The listing builds one solid part. Answer for the finished solid, in the listing's coordinates (mm). Face numbers are marked on the shaded views. A direction names the side the tool comes from. Give positions to 0.01 mm unless a question says otherwise; leave off trailing zeros. Order: outer loops, then holes, each group sorted by start corner. A loop starts at its lowest first (then second) coordinate and runs counter-clockwise, first axis right, second up. Notation, with made-up numbers: (27.25, 60) - (44.25, 60) arc R22 ccw to (44.25, 80) - close; hole circle Ø1 at (-4, 48). An arc over 180 degrees is marked (long way). Answer in a Markdown table with one row per item.
from build123d import *

# Parameters (mm, degrees)
F0_R     = 14.95
F1_DEPTH = 20.6
F2_R     = 12.5
F3_DEPTH = 4
F4_R     = 12.5
F5_DEPTH = 4.5
F6_R     = 5
F7_DEPTH = 25


with BuildPart() as f1:
    # F0 (on Front) → F1 (new body)
    with BuildSketch(Plane.XZ):
        Circle(F0_R)
    extrude(amount=F1_DEPTH)

    # F2 (on face) → F3 (join)
    with BuildSketch(Plane.XZ.offset(20.6)):
        Circle(F2_R)
    extrude(amount=F3_DEPTH)

    # F4 (on face) → F5 (cut)
    with BuildSketch(Plane(origin=(0, 0, 0), x_dir=(-1, 0, 0), z_dir=(0, 1, 0))):
        Circle(F4_R)
    extrude(amount=-F5_DEPTH, mode=Mode.SUBTRACT)

    # F6 (on face) → F7 (cut)
    with BuildSketch(Plane(origin=(0, -4.5, 0), x_dir=(-1, 0, 0), z_dir=(0, 1, 0))):
        Circle(F6_R)
    extrude(amount=-F7_DEPTH, mode=Mode.SUBTRACT)


solid = f1.part
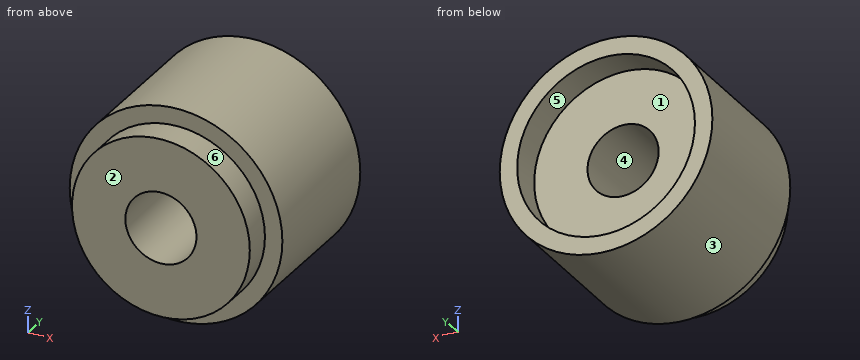
Item 1: Find section B-B on x = 0. Write down the section's boundary in (y, z).
Answer block:
| item | result |
|---|---|
| outline | (-24.6, -12.5) - (-20.6, -12.5) - (-20.6, -14.95) - (0, -14.95) - (0, -12.5) - (-4.5, -12.5) - (-4.5, -5) - (-24.6, -5) - close; (-24.6, 5) - (-4.5, 5) - (-4.5, 12.5) - (0, 12.5) - (0, 14.95) - (-20.6, 14.95) - (-20.6, 12.5) - (-24.6, 12.5) - close |
Item 2: Determine the mould class of the marked faces 1, 2 and 3 for opening direction X: pulls with the +X half, pulls with the -X half, needs draft (parallel to the pull), parting line crosses it, or undercut.
Answer block:
| item | result |
|---|---|
| face 1 | undercut |
| face 2 | needs draft |
| face 3 | parting line crosses it |
Item 3: Consider line 1 (Z direction, x = 0, y = -18.25); line 2 (Y direction, x = -10.5, z = -0.5); line 3 (Y direction, x = -9.5, z = -11). Determine where each line is inside the solid, lowest interval first.
Answer block:
| item | result |
|---|---|
| line 1 | -14.95 to -5, 5 to 14.95 |
| line 2 | -24.6 to -4.5 |
| line 3 | -20.6 to 0 |
Item 4: Find section A-A on z = 0. Write down the section's boundary in (x, y), then the cut area to 3 significant figures.
Answer block:
| item | result |
|---|---|
| outline | (-14.95, -20.6) - (-12.5, -20.6) - (-12.5, -24.6) - (-5, -24.6) - (-5, -4.5) - (-12.5, -4.5) - (-12.5, 0) - (-14.95, 0) - close; (5, -24.6) - (12.5, -24.6) - (12.5, -20.6) - (14.95, -20.6) - (14.95, 0) - (12.5, 0) - (12.5, -4.5) - (5, -4.5) - close |
| area | 402 mm² |
Item 5: Find section C-C on y = -7.5. Write down the section's boundary in (x, z).
Answer block:
| item | result |
|---|---|
| outline | circle Ø29.9 at (0, 0); hole circle Ø10 at (0, 0) |
Item 6: Which of the six approach directions +Z, -Z, +X, -X, +Y, -Y give full straight-line access (tool end or side, diameter ignored) to the marked faces 4, 5 and 6?
Answer block:
| item | result |
|---|---|
| face 4 | +Y, -Y |
| face 5 | +Y |
| face 6 | -Y |
Item 7: Each of these flat-tipped pins is pushed along its axis until it touches: P1, Ø5, axis at x = 10.5, y = -14, coming from the +Z side; P2, Ø3, axis at y = -11.5, z = -6.5, coming from the +X side; P3, Ø12.5, axis at x = 4, z = 3.5, coming from the +Y side. Where does it stop, or does it pass through?
Answer block:
| item | result |
|---|---|
| P1 | z = 12.63 |
| P2 | x = 14.09 |
| P3 | y = -4.5 |
Item 8: Find section D-D on z = 11.75. Write down the section's boundary in (x, y).
Answer block:
| item | result |
|---|---|
| outline | (-9.24, -20.6) - (-4.26, -20.6) - (-4.26, -24.6) - (4.26, -24.6) - (4.26, -20.6) - (9.24, -20.6) - (9.24, 0) - (4.26, 0) - (4.26, -4.5) - (-4.26, -4.5) - (-4.26, 0) - (-9.24, 0) - close |
